```python
from build123d import *

# Parameters (mm, degrees)
SKETCH_1_W          = 38
SKETCH_1_H          = 75
EXTRUDE_1_DEPTH     = 30.73
SKETCH_2_R          = 7.8
EXTRUDE_2_DEPTH     = 7.2
SKETCH_3_W          = 30.7
SKETCH_3_H          = 10.4
EXTRUDE_3_DEPTH     = 6.4
SKETCH_5_W          = 30.5
SKETCH_5_H          = 67
CUT_EXTRUDE_1_DEPTH = 60.648829829
CUT_EXTRUDE_2_REACH = 87.181
SKETCH_6_W          = 9.8
SKETCH_6_H          = 20.33
CUT_EXTRUDE_3_REACH = 69.808
SKETCH_8_R          = 1.4
CUT_EXTRUDE_4_DEPTH = 7.4


with BuildPart() as part:
    # 草图1 → 凸台-拉伸1 (new body)
    with BuildSketch(Plane(origin=(0, 0, 0), x_dir=(1, 0, 0), z_dir=(0, 1, 0))):
        Rectangle(SKETCH_1_W, SKETCH_1_H)
    extrude(amount=EXTRUDE_1_DEPTH)

    # 草图2 → 凸台-拉伸2 (add)
    with BuildSketch(Plane.ZY.offset(19)):
        with Locations(Location((-17.53, 13.39, 0), (0, 0, 180))):
            Circle(SKETCH_2_R)
    extrude_2 = extrude(amount=EXTRUDE_2_DEPTH)

    # 草图3 → 凸台-拉伸3 (add)
    with BuildSketch(Plane(origin=(0, 0, -37.5), x_dir=(-1, 0, 0), z_dir=(0, 0, -1))):
        with Locations((0, 25.53)):
            Rectangle(SKETCH_3_W, SKETCH_3_H)
    extrude_3 = extrude(amount=EXTRUDE_3_DEPTH)

    # 草图5 → 切除-拉伸1 (cut, through all)
    with BuildSketch(Plane(origin=(0, 30.73, 0), x_dir=(1, 0, 0), z_dir=(0, 1, 0))):
        Rectangle(SKETCH_5_W, SKETCH_5_H)
    extrude(amount=-CUT_EXTRUDE_1_DEPTH, mode=Mode.SUBTRACT)

    # 镜向2: 凸台-拉伸2 across plane
    add(extrude_2.mirror(Plane(origin=(0, 0, 0), x_dir=(0, 0, 1), z_dir=(1, 0, 0))))

    # 草图6 → 切除-拉伸2 (cut, up to next)
    with BuildSketch(Plane(origin=(0, 0, -37.5), x_dir=(-1, 0, 0), z_dir=(0, 0, -1)), mode=Mode.PRIVATE) as cut_extrude_2_sk1:
        with Locations((0, 10.165)):
            Rectangle(SKETCH_6_W, SKETCH_6_H)
    cut_extrude_2_tool1 = extrude(cut_extrude_2_sk1.sketch, amount=-CUT_EXTRUDE_2_REACH, mode=Mode.PRIVATE) & part.part
    add(cut_extrude_2_tool1.solids().sort_by_distance((0, 10.165, -37.5))[0], mode=Mode.SUBTRACT)

    # 草图7 → 切除-拉伸3 (cut, up to next)
    with BuildSketch(Plane(origin=(15.35, 0, 0), x_dir=(0, 0, -1), z_dir=(1, 0, 0)), mode=Mode.PRIVATE) as cut_extrude_3_sk1:
        Polygon((37.5, 20.33), (43.9, 25.33022801), (43.9, 20.33), align=None)
    cut_extrude_3_tool1 = extrude(cut_extrude_3_sk1.sketch, amount=-CUT_EXTRUDE_3_REACH, mode=Mode.PRIVATE) & part.part
    cut_extrude_3 = cut_extrude_3_tool1.solids().sort_by_distance((15.35, 21.996743, -41.766667))[0]
    add(cut_extrude_3, mode=Mode.SUBTRACT)

    # 镜向4: 凸台-拉伸3, 切除-拉伸3 across plane
    add(extrude_3.mirror(Plane.XY))
    add(cut_extrude_3.mirror(Plane.XY), mode=Mode.SUBTRACT)

    # 草图8 → 切除-拉伸4 (cut)
    with BuildSketch(Plane(origin=(0, 30.73, 0), x_dir=(1, 0, 0), z_dir=(0, 1, 0))):
        with Locations(Location((-8.5, 37.5, 0), (0, 0, 270))):
            Circle(SKETCH_8_R)
        with Locations(Location((8.5, 37.5, 0), (0, 0, 90))):
            Circle(SKETCH_8_R)
        with Locations(Location((8.5, -37.5, 0), (0, 0, 270))):
            Circle(SKETCH_8_R)
        with Locations(Location((-8.5, -37.5, 0), (0, 0, 90))):
            Circle(SKETCH_8_R)
    extrude(amount=-CUT_EXTRUDE_4_DEPTH, mode=Mode.SUBTRACT)


solid = part.part
```
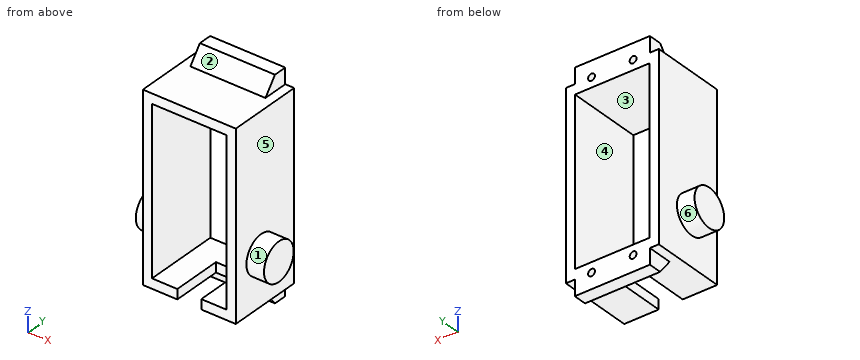
Part model, mm, in its own coordinate system. Face numbers are marked on the shaded views. A direction names the side the tool comes from. Give positions to 0.01 mm unless a question says otherwise; leave off trailing zeros. Write each loop counter-clockwise with the first axis right and the second up, starting at its lowest first coordinate (ties: lowest second). Pieces come first, ordered by that corner, then holes. Notation, with made-up numbers: (37, 40) -> (54, 40) arc R26 ccw to (54, 59) -> close; hole circle Ø7 at (10.25, -29.75). An arc over 180 degrees is marked (long way). Put each result on its own line as item: value. Start each with the question number.
Item 1: Cut at C-C (y = 13.39). List the corners of the cut face in (x, z), then the cut area to 3 significant figures.
Item 2: Cut at B-B (z = -17.53). List the corners of the cut face in (x, y), then the cut area to 3 significant figures.
Item 3: Pull direction X, two halves, no side cores. Call the marked faces 4, 5 and 6: pulls with the +X half, pulls with the -X half, needs draft (parallel to the pull), parting line crosses it, or undercut.
Item 4: Pin check, flat tips, straight feed: pin 1 Ø9 at (y, z) = (22, 14) entering from +X; pin 2 Ø5 at (x, y) = (3, 6) entering from -Z; pin 3 Ø1.9 at (y, z) = (27.5, 40.5) entering from +X; pin 4 Ø12 at (y, z) = (7, -26) entering from -X. Stop position of each tip, or through.
Item 5: Wall check: L1, parallel to X at y = 2, z = -4; L2, parallel to Z at x = 13, y = 19.5; L3, parallel to Z at x = 18.5, y = 3. Give the ranges that are in metal, low to high. Write a range as [from, to].
Item 6: Cut at A-A (x = 8.5). List the corners of the cut face in (y, z).
Item 7: Which spindle directions (+Z, -Z, +X, -X, +Y, -Y) get a long thin tool onto all of the face, cutting with end or side? Do the marked faces 1, 2 and 3. Say none if no direction does.
Item 8: Cut at D-D (z = 24). List the corners of the cut face in (x, y), then the cut area to 3 significant figures.
Answer list:
1. outline: (-26.2, -25.33) -> (-19, -25.33) -> (-19, -37.5) -> (-4.9, -37.5) -> (-4.9, -33.5) -> (-15.25, -33.5) -> (-15.25, 33.5) -> (15.25, 33.5) -> (15.25, -33.5) -> (4.9, -33.5) -> (4.9, -37.5) -> (19, -37.5) -> (19, -25.33) -> (26.2, -25.33) -> (26.2, -9.73) -> (19, -9.73) -> (19, 37.5) -> (-19, 37.5) -> (-19, -9.73) -> (-26.2, -9.73) -> close
1. area: 992 mm2
2. outline: (-26.2, 5.59) -> (-19, 5.59) -> (-19, 0) -> (-15.25, 0) -> (-15.25, 30.73) -> (-19, 30.73) -> (-19, 21.19) -> (-26.2, 21.19) -> close; (15.25, 0) -> (19, 0) -> (19, 5.59) -> (26.2, 5.59) -> (26.2, 21.19) -> (19, 21.19) -> (19, 30.73) -> (15.25, 30.73) -> close
2. area: 455 mm2
3. face 4: undercut
3. face 5: pulls with the +X half
3. face 6: needs draft
4. pin 1: stops at x = 19
4. pin 2: stops at z = -37.5
4. pin 3: stops at x = 15.35
4. pin 4: stops at x = -26.2
5. L1: x = [-19, -15.25], [15.25, 19]
5. L2: z = [-37.5, -33.5], [33.5, 37.5]
5. L3: z = [-37.5, 37.5]
6. outline: (0, -37.5) -> (20.33, -37.5) -> (25.33, -43.9) -> (30.73, -43.9) -> (30.73, -38.9) -> (23.33, -38.9) -> (23.33, -36.1) -> (30.73, -36.1) -> (30.73, -33.5) -> (0, -33.5) -> close; (0, 33.5) -> (30.73, 33.5) -> (30.73, 36.1) -> (23.33, 36.1) -> (23.33, 38.9) -> (30.73, 38.9) -> (30.73, 43.9) -> (25.33, 43.9) -> (20.33, 37.5) -> (0, 37.5) -> close
7. face 1: +X
7. face 2: +Z, +X, -X, -Y
7. face 3: +Y, -Y
8. outline: (-19, 0) -> (-15.25, 0) -> (-15.25, 30.73) -> (-19, 30.73) -> close; (15.25, 0) -> (19, 0) -> (19, 30.73) -> (15.25, 30.73) -> close
8. area: 230 mm2
